Input: part model. Units: mm. Frame: model coordinates. Face numbers are marked on the shaded views. A direction names the side the tool comes from. Round coordinates to 2 decimals unless told otherwise and drop trailing zeros. Loops run counter-clockwise (first coordinate to the right, second up) from the corner with the lowest first, then second, coordinate; pieces in that order, holes last. Notation, with made-up numbers: M -12,0.5 L 35,0.5 A23 ccw 35,9.5 Z; hole C 27,71 d4. An arc over 180 degrees is marked long. Use one line per item in the form item = value. Start each with the question number.
Q1. Mould query, pull axis X, two halves, no side actions, for the marked faces 1 and 2. Classes: pulls with the +X half, pulls with the -X half, needs draft (parallel to the pull), parting line crosses it, or undercut.
Q2. Ray query, line 1 along X through (y, z) = (0.1, 1); line 2 along Z through (x, y) = (1.55, 1.3); line 3 along Y through (x, z) = (-1.65, 3). Return the intervals inside material, ascending.
Q3. Access query for the marked faces 3 and 4. Directions: +Z, -Z, +X, -X, +Y, -Y. A direction counts if a zero-diameter tool reaches every point of the face in a straight line with its end or side. Return the directions, or none.
Q4. First-contact query: P1, Ø1, axis at x = 0, z = -0.5, coming from the -Y side (3 decimals); P2, Ø3, axis at x = 1.5, z = 2, coming from the -Y side; P3, Ø3, axis at y = 1, z = -1, coming from the -X side (3 decimals). Flat tips, straight axial feed; report the tip coordinate or a pass-through.
Q5. Section query C-C, the plane z = 4. Output: boundary loops of the cut face in (x, y).
Q6. Section query D-D, the plane z = 5.25. Output: boundary loops of the cut face in (x, y).
Q7. Section query A-A, the plane y = 0. Output: boundary loops of the cut face in (x, z) (3 decimals).
```python
from build123d import *

# Parameters (mm, degrees)
SKETCH_1_R      = 2.45
EXTRUDE_1_DEPTH = 5
SKETCH_2_R      = 2.5
EXTRUDE_2_DEPTH = 2.25
SKETCH_3_R      = 2.475
EXTRUDE_3_DEPTH = 2.25
FILLET_1_R      = 0.5


with BuildPart() as part:
    # 스케치1 → 보스-돌출1 (new body)
    with BuildSketch(Plane.XY):
        Circle(SKETCH_1_R)
    extrude(amount=EXTRUDE_1_DEPTH)

    # 스케치2 → 보스-돌출2 (add)
    with BuildSketch(Plane.XY.offset(5)):
        Circle(SKETCH_2_R)
    extrude(amount=EXTRUDE_2_DEPTH)

    # 스케치3 → 보스-돌출3 (add)
    with BuildSketch(Plane(origin=(0, 0, 0), x_dir=(-1, 0, 0), z_dir=(0, 0, -1))):
        Circle(SKETCH_3_R)
    extrude(amount=EXTRUDE_3_DEPTH)

    # 필렛1
    fillet_1_edges = [part.edges().sort_by_distance(p)[0] for p in [
        (-2.5, 0, 7.25),
        (2.475, 0, -2.25),
    ]]
    fillet(fillet_1_edges, radius=FILLET_1_R)


solid = part.part
```
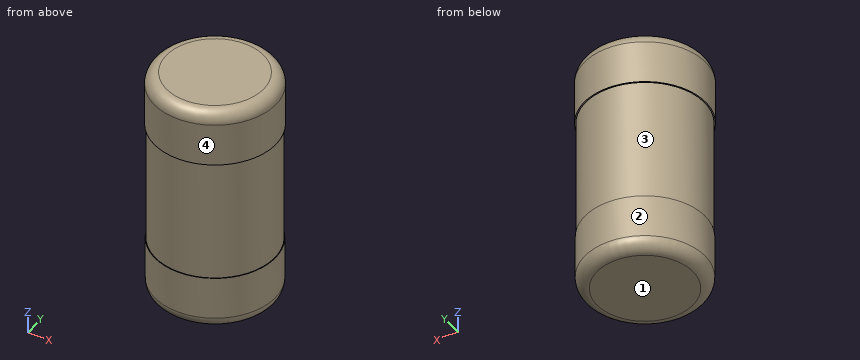
Results found:
q1.face_1 = needs draft
q1.face_2 = parting line crosses it
q2.line_1 = -2.45 to 2.45
q2.line_2 = -2.25 to 7.25
q2.line_3 = -1.81 to 1.81
q3.face_3 = none
q3.face_4 = +Z, -Z
q4.P1 = -2.475
q4.P2 = -2.45
q4.P3 = -2.475
q5.outline = C 0,0 d4.9
q6.outline = C 0,0 d5
q7.outline = M -2.5,5 L -2.45,5 L -2.45,0 L -2.475,0 L -2.475,-1.75 A0.5 ccw -1.975,-2.25 L 1.975,-2.25 A0.5 ccw 2.475,-1.75 L 2.475,0 L 2.45,0 L 2.45,5 L 2.5,5 L 2.5,6.75 A0.5 ccw 2,7.25 L -2,7.25 A0.5 ccw -2.5,6.75 Z
